Design review of the part built by this model. Coordinates are the model's own, in mm. A direction names the side the tool comes from. Coordinates: 2 decimals unless noted, no trailing zeros. Write each loop counter-clockwise with the first axis right and the second up, starting at its lowest first coordinate (ties: lowest second). Pieces come first, ordered by that corner, then holes.
Q1. Take a section at B-B (z = -3.5). Give the boundary of the cut face in (x, y).
Q2. Mouldability with a two-part tool opening along X and no side actions: class faces 1 (the flat face through (12.7, -1, 1)), 2 (the cylindrical face through (15.822, 23.802, 1.174)), 3 (the flat face through (6, -1.276, 1)) as pulls with the +X half, pulls with the -X half, needs draft (parallel to the pull), parting line crosses it, or undercut.
Q3. Machinability: for faces 4 (the cylindrical face through (0.362, -0.647, 7.159)), 5 (the flat face through (11, 11, 2.381)), which of the approach directions +Z, -Z, +X, -X, +Y, -Y give a long, thin tool a straight path to every point of the face, cutting with its end or side? Answer none if there is none.
Q4. Take a section at A-A (x = 8). Give the boundary of the cut face in (y, z), and give its area (3 significant figures).
Q5. Insertion check: pin 1 (8 mm diameter, centred on x = 7.5, y = 17, fed in from +Z); pin 2 (3 mm diameter, centred on x = 5.5, z = 5.5, fed in from +Y); pin 3 (3 mm diameter, centred on x = 7.5, y = 9, fed in from -Z). Each pin has a flat end and moves straight along its axis. Give the tip position at first contact, or say it passes through.
Q6. For probe 1 along Y at (x, z) = (3.25, 5.5); probe 2 along Z at (x, y) = (7.25, 7.75); probe 3 along X at (y, z) = (0.5, 0.25), list the stretches that pass through material, from the lowest coordinate up.
Q7. Take a section at D-D (x = 2.75). Give the boundary of the cut face in (y, z).
Q8. Take a section at C-C (y = 11.75). Give the boundary of the cut face in (x, z).
```python
from build123d import *

# Parameters (mm, degrees)
SKETCH1_R           = 0.5999988
BOSS_EXTRUDE1_DEPTH = 2.38125
SKETCH2_W           = 12.7
SKETCH2_H           = 12.7
BOSS_EXTRUDE2_DEPTH = 1.27635
FILLET1_R           = 1.27


with BuildPart() as part:
    # Sketch1 → Boss-Extrude1 (new body)
    with BuildSketch(Plane.XY):
        with BuildLine():
            Line((0, 0), (13.692383752, 24.509366916))
            ThreePointArc((13.692383752, 24.509366916), (14.330250369, 25.160900132), (15.210137069, 25.4))
            Line((15.210137069, 25.4), (15.289057138, 25.4))
            ThreePointArc((15.289057138, 25.4), (16.518390537, 24.890793433), (17.027597104, 23.661460034))
            Line((17.027597104, 23.661460034), (17.027597104, 4.405539966))
            ThreePointArc((17.027597104, 4.405539966), (16.518390537, 3.176206567), (15.289057138, 2.667))
            Line((15.289057138, 2.667), (15.210137069, 2.667))
            ThreePointArc((15.210137069, 2.667), (14.330250369, 2.427900132), (13.692383752, 1.776366916))
            Line((13.692383752, 1.776366916), (12.7, 0))
            Line((12.7, 0), (0, 0))
        make_face()
        with Locations((15.249597104, 4.445)):
            Circle(SKETCH1_R, mode=Mode.SUBTRACT)
        with Locations((15.249597104, 23.622)):
            Circle(SKETCH1_R, mode=Mode.SUBTRACT)
        with Locations((15.249597104, 14.0335)):
            Circle(SKETCH1_R, mode=Mode.SUBTRACT)
        with Locations((15.249597104, 18.8595)):
            Circle(SKETCH1_R, mode=Mode.SUBTRACT)
        with Locations((15.249597104, 9.2075)):
            Circle(SKETCH1_R, mode=Mode.SUBTRACT)
    extrude(amount=BOSS_EXTRUDE1_DEPTH)

    # Sketch2 → Boss-Extrude2 (add)
    with BuildSketch(Plane.XZ):
        with Locations((6.35, 1.190625)):
            Rectangle(SKETCH2_W, SKETCH2_H)
    extrude(amount=BOSS_EXTRUDE2_DEPTH)

    # Fillet1
    fillet1_edges = [part.edges().sort_by_distance(p)[0] for p in [
        (6.35, 0, 0),
        (6.35, 0, 2.38125),
        (12.7, -0.638175, 7.540625),
        (12.7, -0.638175, -5.159375),
        (0, -0.638175, -5.159375),
        (0, -0.638175, 7.540625),
    ]]
    fillet(fillet1_edges, radius=FILLET1_R)


solid = part.part
```
Response:
1. outline: (0, -1.28) - (12.7, -1.28) - (12.7, 0) - (0, 0) - close
2. face 1: pulls with the +X half
2. face 2: undercut
2. face 3: needs draft
3. face 4: +Z, -X, +Y, -Y
3. face 5: +Z, +X, -X, +Y
4. outline: (-1.28, -5.16) - (0, -5.16) - (0, -1.27) arc R1.27 cw to (1.27, 0) - (14.32, 0) - (14.32, 2.38) - (1.27, 2.38) arc R1.27 cw to (0, 3.65) - (0, 7.54) - (-1.28, 7.54) - close
4. area: 51.0 mm2
5. pin 1: stops at z = 2.38
5. pin 2: stops at y = 0
5. pin 3: stops at z = 0
6. probe 1: y = -1.28 to 0
6. probe 2: z = 0 to 2.38
6. probe 3: x = 0.28 to 12.98
7. outline: (-1.28, -5.16) - (0, -5.16) - (0, -1.27) arc R1.27 cw to (1.27, 0) - (4.92, 0) - (4.92, 2.38) - (1.27, 2.38) arc R1.27 cw to (0, 3.65) - (0, 7.54) - (-1.28, 7.54) - close
8. outline: (6.56, 0) - (17.03, 0) - (17.03, 2.38) - (6.56, 2.38) - close
